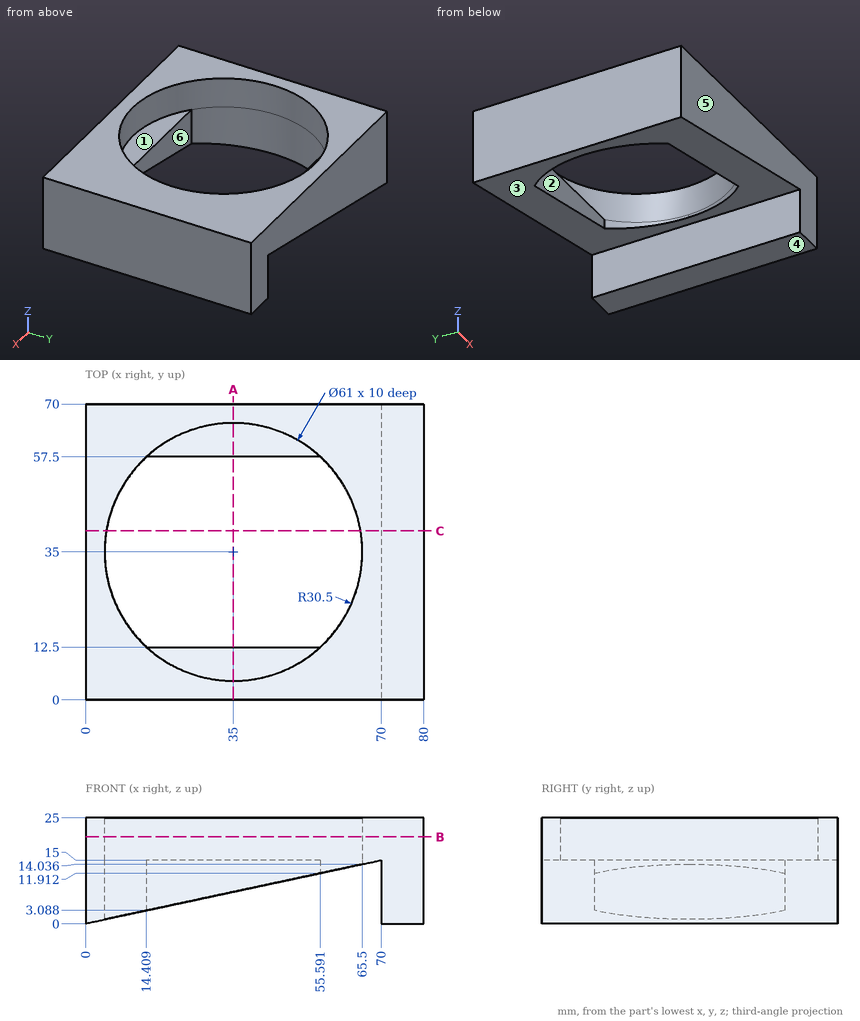
Job drawing, mm, ordinate dimensions from the low corner. One solid piece. A direction names the side the tool comes from. Give positions to 0.01 mm unless a question says otherwise; leave off trailing zeros. Write each loop counter-clockwise with the first axis right and the second up, starting at its lowest first coordinate (ties: lowest second). Pieces come first, ordered by that corner, then holes. Notation, with made-up numbers: M -1,62.25 L 25,62.25 A20 ccw 25,69.25 Z; hole C 25,-25.5 d2. An arc over 180 degrees is marked long. Put each result on its own line as item: value. Start each with the question number.
(1) Mould opens along Y. For the marked faces 4, 5 and 6 say: +Y half, -Y half, draft (parallel to the pull), parting line (faces both ways), or undercut.
(2) Band-saw the part on A-A, the plane x = 35. Write the cut outline in (y, z).
(3) Probe L1, parallel to Y at x = 35, z = 20; L2, parallel to X at y = 34.5, z = 1.25; L3, parallel to Y at x = 24.5, z = 9.25. List the from-to ranges inside material, lowest first.
(4) Flat gauge pins, fed straight in: pin 1 Ø1 at (x, y) = (37, 14.5) entering from -Z; pin 2 Ø4 at (x, y) = (44, 9) entering from +Z; pin 3 Ø10 at (x, y) = (21.5, 10.5) entering from -Z. Where does each tip first touch, or does it go through?
(5) Band-saw the part on B-B, the plane z = 20.5. Write the cut outline in (x, y), and give its area (3 significant figures).
(6) Band-saw the part on C-C, the plane y = 40. Write the cut outline in (x, z).
(7) Which spindle directions (+Z, -Z, +X, -X, +Y, -Y) get a long thin tool onto all of the face, cutting with end or side? Do the marked faces 1, 2 and 3. Say none if no direction does.
Response values:
1. face 4: draft
1. face 5: -Y half
1. face 6: undercut
2. outline: M 0,7.5 L 12.5,7.5 L 12.5,15 L 4.5,15 L 4.5,25 L 0,25 Z; M 57.5,7.5 L 70,7.5 L 70,25 L 65.5,25 L 65.5,15 L 57.5,15 Z
3. L1: y = 0 to 4.5, 65.5 to 70
3. L2: x = 0 to 4.5, 70 to 80
3. L3: y = 0 to 12.5, 57.5 to 70
4. pin 1: passes through
4. pin 2: stops at z = 15
4. pin 3: stops at z = 3.54
5. outline: M 0,0 L 80,0 L 80,70 L 0,70 Z; hole C 35,35 d61
5. area: 2,680 mm2
6. outline: M 0,0 L 4.91,1.05 L 4.91,25 L 0,25 Z; M 65.09,13.95 L 70,15 L 70,0 L 80,0 L 80,25 L 65.09,25 Z
7. face 1: +Z
7. face 2: +Z, -Z
7. face 3: -Z, +Y, -Y
